Read the model definition and answer for the solid it produces. Units are mm, in the model's axes. A direction names the side the tool comes from. Coordinates: 2 decimals unless noted, no trailing zeros. Loops run counter-clockwise (first coordinate to the right, second up) from the corner with the lowest first, then second, coordinate; pieces in that order, holes last.
from build123d import *

# Parameters (mm, degrees)
SKETCH1_R           = 1
SKETCH1_R_2         = 1.5
BOSS_EXTRUDE1_DEPTH = 3


with BuildPart() as part:
    # Sketch1 → Boss-Extrude1 (new body)
    with BuildSketch(Plane.XY):
        with BuildLine():
            Line((-59.247809755, 25.254592271), (-59.247809755, 18.533720681))
            Line((-59.247809755, 18.533720681), (-45.247809755, 18.533720681))
            Line((-45.247809755, 18.533720681), (-45.247809755, -4.966279319))
            Line((-45.247809755, -4.966279319), (-59.247809755, -4.966279319))
            Line((-59.247809755, -4.966279319), (-59.247809755, -8.575462785))
            ThreePointArc((-59.247809755, -8.575462785), (-59.195128163, -9.299369248), (-59.038193528, -10.008021094))
            Line((-59.038193528, -10.008021094), (-52.173270473, -32.963886693))
            ThreePointArc((-52.173270473, -32.963886693), (-51.922175056, -34.097729646), (-51.83788451, -35.255979988))
            Line((-51.83788451, -35.255979988), (-51.83788451, -65.202303041))
            ThreePointArc((-51.83788451, -65.202303041), (-50.943230184, -66.196738704), (-49.860079932, -65.411822033))
            Line((-49.860079932, -65.411822033), (-37.949217773, -9.824997069))
            ThreePointArc((-37.949217773, -9.824997069), (-37.866062344, -9.304130483), (-37.838240661, -8.777402109))
            Line((-37.838240661, -8.777402109), (-37.838240661, 24.285754655))
            ThreePointArc((-37.838240661, 24.285754655), (-37.929542195, 25.236900999), (-38.200112409, 26.153310895))
            Line((-38.200112409, 26.153310895), (-44.217426695, 41.09747953))
            ThreePointArc((-44.217426695, 41.09747953), (-44.495580184, 41.337138252), (-44.852002492, 41.248997433))
            Line((-44.852002492, 41.248997433), (-58.224251279, 29.538573021))
            ThreePointArc((-58.224251279, 29.538573021), (-58.979963171, 28.520742463), (-59.247809755, 27.28165501))
            Line((-59.247809755, 27.28165501), (-59.247809755, 25.254592271))
        make_face()
        with Locations((-52.247809755, 20.533720681)):
            Circle(SKETCH1_R, mode=Mode.SUBTRACT)
        with Locations((-52.247809755, -6.966279319)):
            Circle(SKETCH1_R, mode=Mode.SUBTRACT)
        with Locations((-48.107299335, -37.682543737)):
            Circle(SKETCH1_R_2, mode=Mode.SUBTRACT)
        with Locations((-48.107299335, -42.050855836)):
            Circle(SKETCH1_R_2, mode=Mode.SUBTRACT)
        with BuildLine():
            Line((-46.243433747, 33.726215246), (-43.028458535, 26.576341757))
            ThreePointArc((-43.028458535, 26.576341757), (-43.050168294, 26.290383394), (-43.302070317, 26.153310895))
            Line((-43.302070317, 26.153310895), (-54.174570897, 26.153310895))
            ThreePointArc((-54.174570897, 26.153310895), (-54.453661171, 26.343271723), (-54.379309982, 26.672586766))
            Line((-54.379309982, 26.672586766), (-46.721784613, 33.822460255))
            ThreePointArc((-46.721784613, 33.822460255), (-46.457870892, 33.897290424), (-46.243433747, 33.726215246))
        make_face(mode=Mode.SUBTRACT)
        with BuildLine():
            Line((-48.107299335, -15.436077517), (-44.378825251, -11.707603433))
            ThreePointArc((-44.378825251, -11.707603433), (-44.021262657, -11.657342723), (-43.874375858, -11.987193319))
            Line((-43.874375858, -11.987193319), (-47.853011905, -29.227949523))
            ThreePointArc((-47.853011905, -29.227949523), (-48.135577902, -29.460333147), (-48.432645874, -29.246800218))
            Line((-48.432645874, -29.246800218), (-53.066527122, -13.820853431))
            ThreePointArc((-53.066527122, -13.820853431), (-52.978484336, -13.510290691), (-52.659725089, -13.459366335))
            Line((-52.659725089, -13.459366335), (-48.107299335, -15.436077517))
        make_face(mode=Mode.SUBTRACT)
    extrude(amount=BOSS_EXTRUDE1_DEPTH)


solid = part.part
Item 1: Find the intervals of material crossed by line 1 along X through (y, z) = (-42, 1.65); line 2 along X through (y, z) = (-20, 2.65); line 3 along X through (y, z) = (-1.5, 0.45), in increasing order.
Numbers:
line 1: x = -51.84 to -49.61, -46.61 to -44.84
line 2: x = -56.05 to -51.21, -45.72 to -40.13
line 3: x = -45.25 to -37.84
Item 2: Determine the mould class of faces 4 (the face through (-46, -12, 0)), 5 (the face through (-51.925, -34.082, 1.479)), 6 (the face through (-50.6, 30.2, 1.5)) for opening direction Y: released by +Y, released by -Y, zero draft, split by the parting line, or undercut.
Numbers:
face 4: zero draft
face 5: released by -Y
face 6: undercut
Item 3: Given pin 1 (1.5 mm diameter, centred on y = 6, z = 2, fed in from -X); pin 2 (1.5 mm diameter, centred on y = -34, z = 2, fed in from +X); pin 3 (1.5 mm diameter, centred on x = -48, z = 2, fed in from +Y), each flat-ended and moving along its own axis, determine where each tip first touches the part or whether it passes through.
Numbers:
pin 1: stops at x = -45.25
pin 2: stops at x = -42.97
pin 3: stops at y = 39.15
Item 4: Which of the six approach directions +Z, -Z, +X, -X, +Y, -Y give full straight-line access (tool end or side, diameter ignored) to faces 1 (the face through (-41.167, 33.521, 1.479)), 2 (the face through (-44.66, 30.2, 1.48)), 3 (the face through (-52, -4.966, 1))?
Numbers:
face 1: +Z, -Z, +X, +Y
face 2: +Z, -Z
face 3: +Z, -Z, -X
Item 5: A cutting plane is placed at D-D on x = -41. Determine the outline of the cut face in (y, z), then the cut area to 3 significant figures.
Numbers:
outline: (-24.06, 0) - (33.11, 0) - (33.11, 3) - (-24.06, 3) - close
area: 172 mm2
Item 6: A cutting plane is placed at C-C on y = 10. Determine the outline of the cut face in (x, z).
Numbers:
outline: (-45.25, 0) - (-37.84, 0) - (-37.84, 3) - (-45.25, 3) - close
Item 7: A cutting plane is placed at B-B on z = 1.7. Give the number of separate pieces and of enclosed holes in the cut face, then the cut area to 3 significant figures.
Numbers:
separate pieces: 1
enclosed holes: 6
area: 1,010 mm2
Item 8: A cutting plane is placed at A-A on x = -57.25. Determine the outline of the cut face in (y, z).
Numbers:
outline: (-15.99, 0) - (-4.97, 0) - (-4.97, 3) - (-15.99, 3) - close; (18.53, 0) - (30.39, 0) - (30.39, 3) - (18.53, 3) - close
